Verification items for the finished model (mm, model axes). Face numbers are marked on the shaded views. A direction names the side the tool comes from. Coordinates: 2 decimals unless noted, no trailing zeros. Write each loop counter-clockwise with the first axis right and the second up, starting at its lowest first coordinate (ties: lowest second). Pieces come first, ordered by that corner, then holes. Notation, with made-up numbers: M 6,44.5 L 21,44.5 A28 ccw 21,68.5 Z; hole C 37,-33.5 d3. An arc over 180 degrees is marked long. One line per item, written item: value.
Autodesk Inventor part; units mm, degrees
ref_plane "Work Plane1" through (8.9551, 0, 0) normal (0, 0, 1) x (-1, 0, 0)
ref_plane "YZ Plane" through (0, 0, 0) normal (1, 0, 0) x (0, 1, 0)
ref_plane "XZ Plane" through (0, 0, 0) normal (0, 1, 0) x (-1, 0, 0)
sketch "Sketch1" plane through (0, 0, 0) normal (1, 0, 0) x (0, 1, 0)
  line L0 (-3.1754, 0) -> (-1.5877, 2.75)
  line L1 (-1.5877, 2.75) -> (1.5877, 2.75)
  line L2 (1.5877, 2.75) -> (3.1754, 0)
  line L3 (3.1754, 0) -> (1.5877, -2.75)
  line L4 (1.5877, -2.75) -> (-1.5877, -2.75)
  line L5 (-1.5877, -2.75) -> (-3.1754, 0)
  point P0 (0, 0)
  point P1 (0, 0)
  dimension "d0" = 6.3509
extrude "Body" add sketch "Sketch1" along normal blind 3.1
sketch "Sketch2" plane through (0, 0, 0) normal (-1, 0, 0) x (0, 0, 1)
  line L0 (0, -4.4456) -> (0, 4.4456)
  line L1 (-3.85, 0) -> (3.85, 0)
  point P0 (0, 0)
hole "Thread" at (0, 0, 0) direction (1, 0, 0) diameter 2.459 end through all
chamfer "Chamfer1" distance 0.2706 angle 30 1 edges at (0, 0, -1.2295) measured on face at (0, -1.925, -1.1495)
chamfer "Chamfer2" distance 0.2706 angle 30 1 edges at (3.1, 0, -1.2295) measured on face at (3.1, -1.925, -1.1495)
sketch "Sketch3" plane through (0, 0, 0) normal (0, 0, 1) x (1, 0, 0)
  line L0 (0, 1.5877) -> (0, 3.1754)
  line L1 (0, 3.1754) -> (3.1, 3.1754)
  line L2 (3.1, 1.5877) -> (3.1, 3.1754)
  line L3 (-0.62, 0) -> (3.72, 0)
  line L4 (0.2456, 3.1754) -> (0, 2.75)
  line L5 (3.1, 2.3375) -> (2.3986, 2.3375)
  line L6 (2.3986, 2.3375) -> (1.4, 3.1754)
  dimension "d3" = 30
  dimension "d5" = 5.5
  dimension "d6" = 4.675
  dimension "d8" = 50
  dimension "d9" = 1.4
revolve "Chamfer3" cut sketch "Sketch3" angle 360 about axis through (-10, 0, 0) along (1, 0, 0)
ref_plane "Work Plane1" through (8.9551, 0, 0) normal (0, 0, 1) x (-1, 0, 0)
equation "\"d0\" = 1.1547 * SW"
equation "\"d1\" = KOH"
equation "\"d3\" = ANG1"
equation "\"d5\" = SW0"
equation "\"d6\" = SW1"
equation "\"d8\" = ANG2"
equation "\"d9\" = KOH1"
equation "\"d10\" = -0.5 * GD1 + 0.5 * NND"
equation "\"d39\" = -0.5 * GD1 + 0.5 * NND"
equation "\"d12\" = -0.5 * GD1 + 0.5 * NND"
equation "\"d40\" = -0.5 * GD1 + 0.5 * NND"
equation "\"ANG1\" = 30deg"
equation "\"ANG2\" = 50deg"
equation "\"NND\" = 3"
equation "\"KOH\" = 3.1"
equation "\"SW\" = 5.5"
equation "\"SW0\" = SW"
equation "\"SW1\" = 0.85 * SW"
equation "\"KOH1\" = 1.4"
equation "\"GUL\" = 0.541266 * PTC"
equation "\"THREADDIA\" = 3"
equation "\"TOA\" = 30deg"
equation "\"PTC\" = 0.5"
equation "\"E0\" = 1.155 * SW"
equation "\"GAL\" = 0.541266 * PTC"
properties part number "ANSI B18.16.3M - Property Class 5 and 10 - Metric M3 x 0.5 Metal Type" material "Steel, Mild"
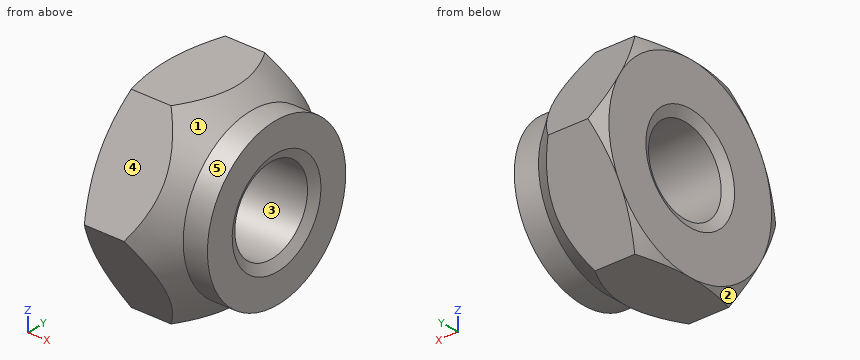
Item 1: Access from +Z, -Z, +X, -X, +Y, -Y to the whole of each face (thin tool, end or side, straight path). Record for the marked faces 4 and 5.
The answers:
face 4: +Z, +X, -X, -Y
face 5: +X
Item 2: Draft check along Z on the marked faces 1, 2 and 3. Enter one of: released by +Z, released by -Z, zero draft, split by the parting line, or undercut.
The answers:
face 1: split by the parting line
face 2: released by -Z
face 3: undercut
Item 3: Scan lines: line 1 (Z direction, x = 1.25, y = 0); line 2 (Y direction, x = 1.5, z = 0); line 3 (Y direction, x = 2.2, z = 0). Record each from-to range of solid material in increasing order.
The answers:
line 1: z = -2.75 to -1.23, 1.23 to 2.75
line 2: y = -3.09 to -1.23, 1.23 to 3.09
line 3: y = -2.5 to -1.23, 1.23 to 2.5
Item 4: Cross-section at A-A, the plane x = 1.3. Enter the section's corners in (y, z).
The answers:
outline: M -3.18,0 L -1.59,-2.75 L 1.59,-2.75 L 3.18,0 L 1.59,2.75 L -1.59,2.75 Z; hole C 0,0 d2.46
